Build history of the part. All positions in model axes, mm. Face numbers are marked on the shaded views. A direction names the side the tool comes from. Round coordinates to 2 decimals unless told otherwise and drop trailing zeros. Order: outer loops, then holes, each group sorted by start corner. A loop starts at its lowest first (then second) coordinate and runs counter-clockwise, first axis right, second up. Notation, with made-up numbers: M -19,-5 L 9,-5 A27 ccw 9,16 Z; hole C -6.75,2.5 d9. An arc over 180 degrees is marked long. One line per item, written item: value. Start each with the question number.
Item 1: Tool access for the marked faces 4, 5, 6, 7 and 8: list every direction of +Z, -Z, +X, -X, +Y, -Y with a clear straight run to the whole face (end or side of a thin tool).
Item 2: Band-saw the part on A-A, the plane y = 0. Write the cut outline in (x, z), then the cut area to 4 significant figures.
Item 3: Band-saw the part on D-D, the plane x = -6.5. Write the cut outline in (y, z).
Item 4: Probe L1, parallel to Y at x = 0, z = 3; L2, parallel to Y at x = 10, z = 9; L3, parallel to Z at x = 9, y = -9. List the from-to ranges inside material, lowest first.
Item 5: Two-plate mould, pull along X, no slides. Class the marked faces 1, 2 and 3: +X half, -X half, draft (parallel to the pull), parting line (faces both ways), or undercut.
Item 6: Pin check, flat tips, straight feed: pin 1 (3.5 mm diameter, centred on x = -7.5, z = 6.5, fed in from +Y); pin 2 (4 mm diameter, centred on x = 23, z = 4, fed in from +Y); pin 3 (1.8 mm diameter, centred on x = 26.5, z = 3.5, fed in from -Y); pin 4 (1.5 mm diameter, centred on x = 21.5, y = -5, fed in from -Z). Stop position of each tip, or through.
Item 7: Band-saw the part on C-C, the plane z = -0.5. Write the cut outline in (x, y).
Item 8: Band-saw the part on B-B, the plane x = 0.5. Write the cut outline in (y, z), then the cut area to 3 significant figures.
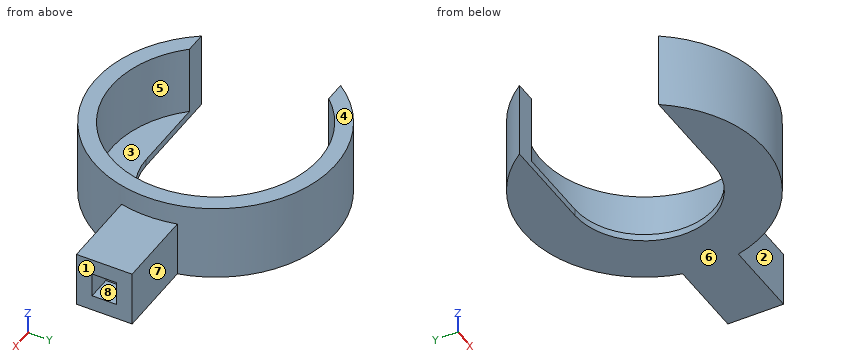
```python
from build123d import *

# Parameters (mm, degrees)
SKETCH1_R                = 17.25
SKETCH1_R_2              = 14.9
BOSS_EXTRUDE1_DEPTH      = 10
BOSS_EXTRUDE3_START      = 1
SKETCH2_R                = 17.25
SKETCH2_R_2              = 10
BOSS_EXTRUDE3_DEPTH      = 1
SKETCH3_R                = 10
CUT_EXTRUDE1_DEPTH       = 27.760511953
BOSS_EXTRUDE4_DEPTH      = 11
BOSS_EXTRUDE4_DEPTH_BACK = 1.5
SKETCH4_W                = 3.5
SKETCH4_H                = 3.5
CUT_EXTRUDE2_DEPTH       = 3.5


with BuildPart() as part:
    # Sketch1 → Boss-Extrude1 (new body)
    with BuildSketch(Plane.XY):
        Circle(SKETCH1_R)
        Circle(SKETCH1_R_2, mode=Mode.SUBTRACT)
    extrude(amount=BOSS_EXTRUDE1_DEPTH)

    # Sketch2 → Boss-Extrude3 (add)
    with BuildSketch(Plane(origin=(0, 0, 0), x_dir=(-1, 0, 0), z_dir=(0, 0, -1)).offset(BOSS_EXTRUDE3_START)):
        Circle(SKETCH2_R)
        Circle(SKETCH2_R_2, mode=Mode.SUBTRACT)
    extrude(amount=-BOSS_EXTRUDE3_DEPTH)

    # Sketch3 → Cut-Extrude1 (cut, through all)
    with BuildSketch(Plane(origin=(0, 0, -1), x_dir=(-1, 0, 0), z_dir=(0, 0, -1))):
        Circle(SKETCH3_R)
        with BuildLine():
            Line((14.055692797, 10), (0, 10))
            ThreePointArc((0, 10), (7.071067812, 7.071067812), (10, 0))
            ThreePointArc((10, 0), (7.071067812, -7.071067812), (0, -10))
            Line((0, -10), (14.055692797, -10))
            ThreePointArc((14.055692797, -10), (16.432029709, -5.248895086), (17.25, 0))
            ThreePointArc((17.25, 0), (16.432029709, 5.248895086), (14.055692797, 10))
        make_face()
    extrude(amount=-CUT_EXTRUDE1_DEPTH, mode=Mode.SUBTRACT)

    # 3DSketch1 → Boss-Extrude4 (add, two sides: drawn at the far end of the back side and taken through both)
    with BuildSketch(Plane(origin=(17.25, 0, -1), x_dir=(0, 0.4472135954999581, 0.8944271909999159), z_dir=(1, 0, 0)).offset(-BOSS_EXTRUDE4_DEPTH_BACK)):
        Polygon((0, 0), (-1.788854382, 3.577708764), (5.366563146, 7.155417528), (8.94427191, 0), (1.788854382, -3.577708764), align=None)
    extrude(amount=BOSS_EXTRUDE4_DEPTH + BOSS_EXTRUDE4_DEPTH_BACK)

    # Sketch4 → Cut-Extrude2 (cut)
    with BuildSketch(Plane(origin=(28.25, 0, 0), x_dir=(0, 0, -1), z_dir=(1, 0, 0))):
        with Locations((-3, 0)):
            Rectangle(SKETCH4_W, SKETCH4_H)
    extrude(amount=-CUT_EXTRUDE2_DEPTH, mode=Mode.SUBTRACT)


solid = part.part
```
Output:
1. face 4: +Z, +X, -X, +Y, -Y
1. face 5: +Z
1. face 6: -Z, +X, -X, +Y, -Y
1. face 7: +Z, -Z, +X, +Y
1. face 8: +X
2. outline: M 10,-1 L 28.25,-1 L 28.25,1.25 L 24.75,1.25 L 24.75,4.75 L 28.25,4.75 L 28.25,7 L 17.25,7 L 17.25,10 L 14.9,10 L 14.9,0 L 10,0 Z
2. area: 106.5 mm²
3. outline: M -15.98,-1 L -10,-1 L -10,0 L -13.41,0 L -13.41,10 L -15.98,10 Z; M 10,-1 L 15.98,-1 L 15.98,10 L 13.41,10 L 13.41,0 L 10,0 Z
4. L1: y = -17.25 to -14.9, 14.9 to 17.25
4. L2: y = -14.06 to -11.05, 11.05 to 14.06
4. L3: z = -1 to 0
5. face 1: +X half
5. face 2: draft
5. face 3: undercut
6. pin 1: stops at y = 16.26
6. pin 2: stops at y = 4
6. pin 3: stops at y = -4
6. pin 4: passes through
7. outline: M -14.06,-10 A17.25 ccw 16.78,-4 L 28.25,-4 L 28.25,4 L 16.78,4 A17.25 ccw -14.06,10 L 0,10 A10 cw 0,-10 Z
8. outline: M -17.24,-1 L -9.99,-1 L -9.99,0 L -14.89,0 L -14.89,10 L -17.24,10 Z; M 9.99,-1 L 17.24,-1 L 17.24,10 L 14.89,10 L 14.89,0 L 9.99,0 Z
8. area: 61.5 mm²
